Can you work these out from the model? Positions are in its coordinate system, mm. A direction names the side the tool comes from. Give positions to 0.01 mm unless a question says otherwise; leave off trailing zeros. Loops run counter-clockwise (first coordinate to the right, second up) from the corner with the lowest first, then second, coordinate; pieces in that order, holes last. Notation, with made-up numbers: (-34.75, 45.5) - (15.25, 45.5) arc R20 ccw to (15.25, 81.5) - close; hole circle Ø2 at (26.5, 34.5). An arc over 180 degrees is marked (long way). Answer as a JSON object with one key per item and string values. Group by question number.
Item 1: Please list where these lines run through material, in increasing order: L1, parallel to Y at x = -3.75, z = 0.85; L2, parallel to Y at x = 0, z = 2.15; L3, parallel to Y at x = -3.5, z = 0.9.
Item 2: Suppose I cut it at D-D on y = 3.25. Write out the boundary of the cut face in (x, z).
Item 3: Suppose I cut it at B-B on x = 0. Write out the boundary of the cut face in (y, z), and give its area (3 significant figures).
Item 4: Suppose I cut it at C-C on x = -3.75. Write out the boundary of the cut face in (y, z), and give its area (3 significant figures).
Item 5: Thinking about a two-plate mould opening in Y: for faces 3 (the cylindrical face through (-1.08, -4.88, 1.48)), 4 (the flat face through (2, 5, 3)), 5 (the cylindrical face through (10, 0, 1)), which applies, pulls with the +Y half, pulls with the -Y half, needs draft (parallel to the pull), parting line crosses it, or undercut?
Item 6: Which directions (+Z, -Z, +X, -X, +Y, -Y) give clear straight access to the entire face, cutting with the end or side of a thin tool? Please do faces 1 (the cylindrical face through (6.7, -0.6, 1.5)), 2 (the flat face through (-8, -3, 1)).
Item 7: Will these pins go through, and if not, where does the flat tip stop? pin 1 (1 mm diameter, centred on y = 1, z = 1.5, fed in from +X); pin 2 (2.5 mm diameter, centred on x = -3.75, y = 6.5, fed in from -Z); pin 3 (0.9 mm diameter, centred on x = -7, z = 1, fed in from -Y); pin 4 (1 mm diameter, centred on y = 7.5, z = 2, fed in from -X).
Item 8: Suppose I cut it at A-A on y = 0. Write out the boundary of the cut face in (x, z), and give its area (3 significant figures).
from build123d import *

# Parameters (mm, degrees)
CROQUIS1_R              = 1
CROQUIS1_R_2            = 5
SALIENTE_EXTRUIR1_DEPTH = 3


with BuildPart() as part:
    # Croquis1 → Saliente-Extruir1 (new body)
    with BuildSketch(Plane.XY):
        with BuildLine():
            Line((-9.539392014, 3), (-6, 3))
            Line((-6, 3), (-6, -3))
            Line((-6, -3), (-9.539392014, -3))
            ThreePointArc((-9.539392014, -3), (10, 0), (-9.539392014, 3))
        make_face()
        with Locations((-3.75, -6.495190528)):
            Circle(CROQUIS1_R, mode=Mode.SUBTRACT)
        with Locations((7.5, 0)):
            Circle(CROQUIS1_R, mode=Mode.SUBTRACT)
        Circle(CROQUIS1_R_2, mode=Mode.SUBTRACT)
        with Locations((-3.75, 6.495190528)):
            Circle(CROQUIS1_R, mode=Mode.SUBTRACT)
    extrude(amount=SALIENTE_EXTRUIR1_DEPTH)


solid = part.part
Worked out:
{
 "1": {"L1": "y = -9.27 to -7.5, -5.5 to -3.31, 3.31 to 5.5, 7.5 to 9.27", "L2": "y = -10 to -5, 5 to 10", "L3": "y = -9.37 to -7.46, -5.53 to -3.57, 3.57 to 5.53, 7.46 to 9.37"},
 "2": {"outline": "(-9.46, 0) - (-3.8, 0) - (-3.8, 3) - (-9.46, 3) - close; (3.8, 0) - (9.46, 0) - (9.46, 3) - (3.8, 3) - close"},
 "3": {"outline": "(-10, 0) - (-5, 0) - (-5, 3) - (-10, 3) - close; (5, 0) - (10, 0) - (10, 3) - (5, 3) - close", "area": "30.0 mm2"},
 "4": {"outline": "(-9.27, 0) - (-7.5, 0) - (-7.5, 3) - (-9.27, 3) - close; (-5.5, 0) - (-3.31, 0) - (-3.31, 3) - (-5.5, 3) - close; (3.31, 0) - (5.5, 0) - (5.5, 3) - (3.31, 3) - close; (7.5, 0) - (9.27, 0) - (9.27, 3) - (7.5, 3) - close", "area": "23.8 mm2"},
 "5": {"face 3": "undercut", "face 4": "needs draft", "face 5": "parting line crosses it"},
 "6": {"face 1": "+Z, -Z", "face 2": "+Z, -Z, -X"},
 "7": {"pin 1": "stops at x = 9.99", "pin 2": "stops at z = 0", "pin 3": "stops at y = -7.56", "pin 4": "stops at x = -7.14"},
 "8": {"outline": "(-6, 0) - (-5, 0) - (-5, 3) - (-6, 3) - close; (5, 0) - (6.5, 0) - (6.5, 3) - (5, 3) - close; (8.5, 0) - (10, 0) - (10, 3) - (8.5, 3) - close", "area": "12.0 mm2"}
}
